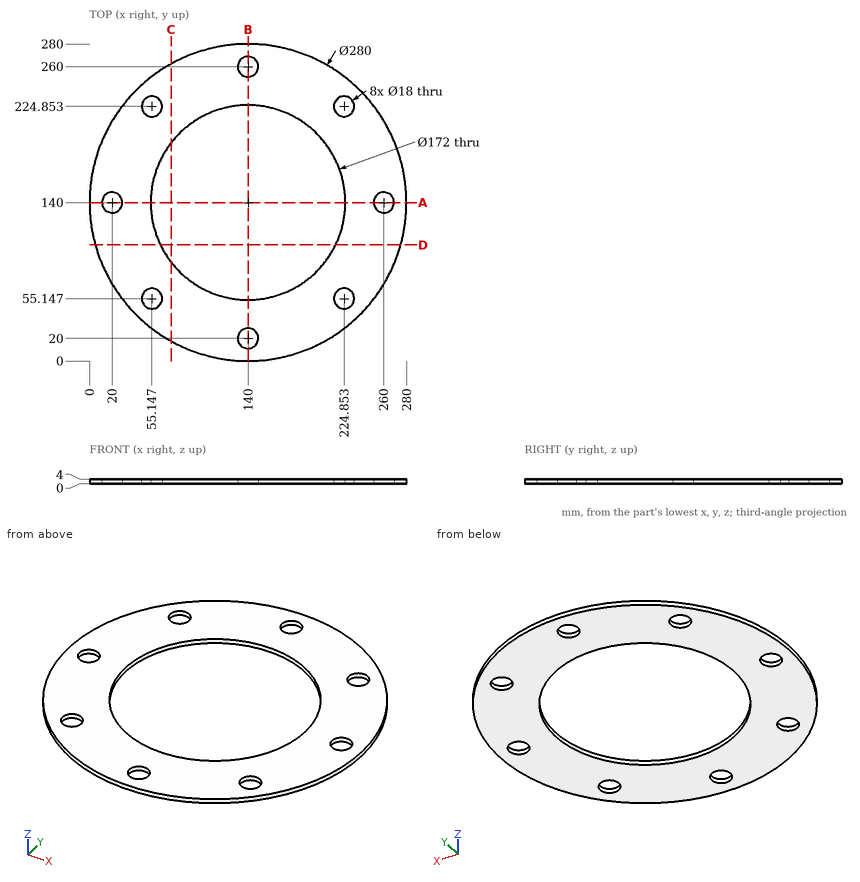
For this review, use the dimensioned drawing (mm, ordinates from the lowest corner) and the shaded views. Coordinates: 2 decimals unless noted, no trailing zeros. Write each loop counter-clockwise with the first axis right and the second up, starting at its lowest first coordinate (ties: lowest second). Pieces come first, ordered by that corner, then holes. Notation, with made-up numbers: (-26, -13) - (2, -13) arc R16 cw to (2, -1) - close; hole circle Ø4 at (22, 83). An arc over 180 degrees is marked (long way). One line per item, written item: value.
1) To check wall thickness, follow probe 1 along X at (y, z) = (141, 1.4); probe 2 along X at (y, z) = (62, 2.8); probe 3 along Y at (x, z) = (89.5, 1.7) (1 decimal). State the ranges of each line that lie inside material, in increasing order.
Answer sheet:
probe 1: x = 0 to 11.06, 28.94 to 54.01, 225.99 to 251.06, 268.94 to 280
probe 2: x = 23.74 to 49.31, 60.98 to 103.78, 176.22 to 219.02, 230.69 to 256.26
probe 3: y = 9.4 to 70.4, 209.6 to 270.6
2) Add section A-A (y = 140). State the section outline as (x, z) points.
Answer sheet:
outline: (0, 0) - (11, 0) - (11, 4) - (0, 4) - close; (29, 0) - (54, 0) - (54, 4) - (29, 4) - close; (226, 0) - (251, 0) - (251, 4) - (226, 4) - close; (269, 0) - (280, 0) - (280, 4) - (269, 4) - close
3) Insertion check: pin 1 (1.5 mm diameter, centred on y = 198.5, z = 1, fed in from +X). The pin has a flat end and moves straight along its axis. Give the tip position at first contact, or say it passes through.
Answer sheet:
pin 1: stops at x = 267.53
4) Add section C-C (x = 72). State the section outline as (y, z) points, plus the area to 3 significant figures.
Answer sheet:
outline: (17.62, 0) - (87.35, 0) - (87.35, 4) - (17.62, 4) - close; (192.65, 0) - (262.38, 0) - (262.38, 4) - (192.65, 4) - close
area: 558 mm2
5) Add section D-D (y = 102.5). State the section outline as (x, z) points.
Answer sheet:
outline: (5.12, 0) - (62.61, 0) - (62.61, 4) - (5.12, 4) - close; (217.39, 0) - (274.88, 0) - (274.88, 4) - (217.39, 4) - close
